CAD build for the part. Positions are in the model's coordinates, mm. A direction names the side the tool comes from. Round coordinates to 2 decimals unless told otherwise and drop trailing zeros. Loops run counter-clockwise (first coordinate to the right, second up) from the corner with the lowest first, then second, coordinate; pieces in that order, holes last.
from build123d import *

# Parameters (mm, degrees)
SKETCH1_W           = 28
SKETCH1_H           = 28
SKETCH1_W_2         = 20
SKETCH1_H_2         = 20
BOSS_EXTRUDE1_DEPTH = 40
SKETCH2_R           = 2.25
CUT_EXTRUDE1_DEPTH  = 30
SKETCH5_W           = 50
SKETCH5_H           = 50
SKETCH5_R           = 1.8
SKETCH5_R_2         = 15
BOSS_EXTRUDE2_DEPTH = 4
SKETCH6_W           = 24
SKETCH6_H           = 28
CUT_EXTRUDE2_DEPTH  = 40
SKETCH7_W           = 4
SKETCH7_H           = 36
CUT_EXTRUDE3_DEPTH  = 4
SKETCH8_W           = 15
SKETCH8_H           = 36
BOSS_EXTRUDE3_DEPTH = 4
BOSS_EXTRUDE4_START = 4
SKETCH11_W          = 50
SKETCH11_H          = 86
SKETCH11_R          = 1.8
SKETCH11_R_2        = 15
SKETCH11_R_3        = 2.25
BOSS_EXTRUDE4_DEPTH = 4
SKETCH13_W          = 8
SKETCH13_H          = 86
BOSS_EXTRUDE5_DEPTH = 2
SKETCH14_W          = 8
SKETCH14_H          = 86
BOSS_EXTRUDE6_DEPTH = 2
SKETCH16_W          = 30
SKETCH16_H          = 86
BOSS_EXTRUDE7_DEPTH = 5


with BuildPart() as part:
    # Sketch1 → Boss-Extrude1 (new body)
    with BuildSketch(Plane(origin=(0, 0, 0), x_dir=(1, 0, 0), z_dir=(0, 1, 0))):
        Rectangle(SKETCH1_W, SKETCH1_H)
        Rectangle(SKETCH1_W_2, SKETCH1_H_2, mode=Mode.SUBTRACT)
    extrude(amount=BOSS_EXTRUDE1_DEPTH)

    # Sketch2 → Cut-Extrude1 (cut)
    with BuildSketch(Plane.ZY.offset(14)):
        with Locations((0, 32)):
            Circle(SKETCH2_R)
        with Locations((0, 16)):
            Circle(SKETCH2_R)
    extrude(amount=-CUT_EXTRUDE1_DEPTH, mode=Mode.SUBTRACT)

    # Sketch5 → Boss-Extrude2 (add)
    with BuildSketch(Plane.ZY.offset(14)):
        with Locations((0, -21)):
            Rectangle(SKETCH5_W, SKETCH5_H)
        with Locations((-15.499780644, -5.500219356)):
            Circle(SKETCH5_R, mode=Mode.SUBTRACT)
        with Locations((15.499780644, -5.500219356)):
            Circle(SKETCH5_R, mode=Mode.SUBTRACT)
        with Locations((15.499780644, -36.499780644)):
            Circle(SKETCH5_R, mode=Mode.SUBTRACT)
        with Locations((-15.499780644, -36.499780644)):
            Circle(SKETCH5_R, mode=Mode.SUBTRACT)
        with Locations((0, -21)):
            Circle(SKETCH5_R_2, mode=Mode.SUBTRACT)
    extrude(amount=-BOSS_EXTRUDE2_DEPTH)

    # Sketch6 → Cut-Extrude2 (cut)
    with BuildSketch(Plane.XZ):
        with Locations((2, 0)):
            Rectangle(SKETCH6_W, SKETCH6_H)
    extrude(amount=-CUT_EXTRUDE2_DEPTH, mode=Mode.SUBTRACT)

    # Sketch7 → Cut-Extrude3 (cut)
    with BuildSketch(Plane.ZY.offset(14)):
        with Locations((-12, 22)):
            Rectangle(SKETCH7_W, SKETCH7_H)
        with Locations((12, 22)):
            Rectangle(SKETCH7_W, SKETCH7_H)
    extrude(amount=-CUT_EXTRUDE3_DEPTH, mode=Mode.SUBTRACT)

    # Sketch8 → Boss-Extrude3 (add)
    with BuildSketch(Plane.ZY.offset(14)):
        with Locations((-17.5, 22)):
            Rectangle(SKETCH8_W, SKETCH8_H)
        with Locations((17.5, 22)):
            Rectangle(SKETCH8_W, SKETCH8_H)
    extrude(amount=-BOSS_EXTRUDE3_DEPTH)

    # Sketch11 → Boss-Extrude4 (add)
    with BuildSketch(Plane.ZY.offset(14).offset(BOSS_EXTRUDE4_START)):
        with Locations((0, -3)):
            Rectangle(SKETCH11_W, SKETCH11_H)
        with Locations((15.499780644, -5.500219356)):
            Circle(SKETCH11_R, mode=Mode.SUBTRACT)
        with Locations((15.499780644, -36.499780644)):
            Circle(SKETCH11_R, mode=Mode.SUBTRACT)
        with Locations((-15.499780644, -36.499780644)):
            Circle(SKETCH11_R, mode=Mode.SUBTRACT)
        with Locations((0, -21)):
            Circle(SKETCH11_R_2, mode=Mode.SUBTRACT)
        with Locations((0, 32)):
            Circle(SKETCH11_R_3, mode=Mode.SUBTRACT)
        with Locations((0, 16)):
            Circle(SKETCH11_R_3, mode=Mode.SUBTRACT)
        with Locations((-15.499780644, -5.500219356)):
            Circle(SKETCH11_R, mode=Mode.SUBTRACT)
    extrude(amount=-BOSS_EXTRUDE4_DEPTH)

    # Sketch13 → Boss-Extrude5 (add)
    with BuildSketch(Plane.XY.offset(25)):
        with Locations((-14, -3)):
            Rectangle(SKETCH13_W, SKETCH13_H)
    extrude(amount=BOSS_EXTRUDE5_DEPTH)

    # Sketch14 → Boss-Extrude6 (add)
    with BuildSketch(Plane(origin=(0, 0, -25), x_dir=(-1, 0, 0), z_dir=(0, 0, -1))):
        with Locations((14, -3)):
            Rectangle(SKETCH14_W, SKETCH14_H)
    extrude(amount=BOSS_EXTRUDE6_DEPTH)

    # Sketch16 → Boss-Extrude7 (add)
    with BuildSketch(Plane(origin=(0, 0, -27), x_dir=(-1, 0, 0), z_dir=(0, 0, -1))):
        with Locations((33, -3)):
            Rectangle(SKETCH16_W, SKETCH16_H)
    boss_extrude7 = extrude(amount=-BOSS_EXTRUDE7_DEPTH)

    # Mirror1: Boss-Extrude7 across plane
    add(boss_extrude7.mirror(Plane.XY))


solid = part.part
Item 1: Flat gauge pin, fed straight in: P1, Ø3, axis at y = -30.5, z = -15.5, coming from the -X side. Where does the tip first touch, or does it go through?
Verdict:
P1: stops at x = -18
Item 2: Mould opens along Z. For faces 3 (the flat face through (-29, -2, -27)), 4 (the flat face through (-18, -4, 0)), 5 (the flat face through (-10, -4, 0)) say: released by +Z, released by -Z, zero draft, split by the parting line, or undercut.
Verdict:
face 3: released by -Z
face 4: undercut
face 5: zero draft
Item 3: Wall check: L1, parallel to Y at x = -14, z = 0; L2, parallel to Z at x = -40, y = 0.5; L3, parallel to X at y = 14, z = -12.5. Give the ranges that are in metal, low to high.
Verdict:
L1: y = -46 to -36, -6 to 13.75, 18.25 to 29.75, 34.25 to 40
L2: z = -27 to -22, 22 to 27
L3: x = -18 to -10
Item 4: Cut at B-B (x = -24). List the corners of the cut face in (y, z), plus the area to 3 significant figures.
Verdict:
outline: (-46, -27) - (40, -27) - (40, -22) - (-46, -22) - close; (-46, 22) - (40, 22) - (40, 27) - (-46, 27) - close
area: 860 mm2
Item 5: Cut at A-A (y = -21). List the corners of the cut face in (x, z), plus the area to 3 significant figures.
Verdict:
outline: (-48, -27) - (-10, -27) - (-10, -15) - (-18, -15) - (-18, -22) - (-48, -22) - close; (-48, 22) - (-18, 22) - (-18, 15) - (-10, 15) - (-10, 27) - (-48, 27) - close
area: 492 mm2
Item 6: Cut at C-C (z = 0). List the corners of the cut face in (x, y).
Verdict:
outline: (-18, -46) - (-10, -46) - (-10, -36) - (-18, -36) - close; (-18, -6) - (-10, -6) - (-10, 13.75) - (-18, 13.75) - close; (-18, 18.25) - (-10, 18.25) - (-10, 29.75) - (-18, 29.75) - close; (-18, 34.25) - (-10, 34.25) - (-10, 40) - (-18, 40) - close
Item 7: Cut at D-D (z = 6.5). List the corners of the cut face in (x, y), plus the area to 3 significant figures.
Verdict:
outline: (-18, -46) - (-10, -46) - (-10, -34.52) - (-18, -34.52) - close; (-18, -7.48) - (-10, -7.48) - (-10, 40) - (-18, 40) - close
area: 472 mm2
Item 8: 3-axis set-ups, long thin cutter, end or side, ignore diameter. For faces 1 (the flat face through (-33, -2, -22)), 2 (the cylindrical face through (-14.056, -35.643, -3.252)): which of +Z, -Z, +X, -X, +Y, -Y reach the whole face in a straight line?
Verdict:
face 1: -X, +Y, -Y
face 2: +X, -X
